For this review, take the finished solid that the model builds, in its own axes (mm). A direction names the side the tool comes from. Coordinates: 2 decimals unless noted, no trailing zeros. Write each loop counter-clockwise with the first axis right and the second up, starting at its lowest first coordinate (ties: lowest second). Pieces come first, ordered by that corner, then holes. Notation, with made-up numbers: M 40.25,-32.75 L 74.25,-32.75 A18 ccw 74.25,-17.75 Z; hole C -35.5,-10.75 d7. An arc over 180 degrees is marked long. Return JSON: item names as keys, results as strings.
```python
from build123d import *

# Parameters (mm, degrees)
F2_R     = 3.81
F3_R     = 5.5372
F4_DEPTH = 177.8


with BuildPart() as f1:
    # F0 (on Front) → F1 (revolve)
    with BuildSketch(Plane.XZ):
        Polygon((0, 6.35), (0, 0), (11.811, 0), (12.7, 12.192), (12.446, 12.192), (10.922, 6.35), align=None)
    revolve(axis=Axis((0, 0, 3.175), (0, 0, -1)))

    # F2
    f2_edges = [f1.edges().sort_by_distance(p)[0] for p in [
        (-11.811, 0, 0),
    ]]
    fillet(f2_edges, radius=F2_R)

    # F3 (on face) → F4 (join)
    with BuildSketch(Plane(origin=(0, 0, 0), x_dir=(1, 0, 0), z_dir=(0, 0, -1))):
        Circle(F3_R)
    extrude(amount=F4_DEPTH)


solid = f1.part
```
1. Clearance check with flat-ended pins moving along their axes: pin 1 Ø8 at (y, z) = (7, -81.5) entering from +X; pin 2 Ø2 at (y, z) = (4, -148) entering from -X; pin 3 Ø1.5 at (x, y) = (8.5, -1.5) entering from +Z; pin 4 Ø8 at (x, y) = (-9.5, -6) entering from +Z. State where each tip first meets the part, or that it passes through.
Checks:
{"pin 1": "x = 4.65", "pin 2": "x = -4.65", "pin 3": "z = 6.35", "pin 4": "z = 12.19"}
2. We need section C-C (z = -136.5). State the section outline as (x, y) points.
Checks:
{"outline": "C 0,0 d11.07"}
3. We need section A-A (y = 0). State the section outline as (x, z) points, plus the area to 3 significant figures.
Checks:
{"outline": "M -12.7,12.19 L -12.07,3.53 A3.81 ccw -8.27,0 L -5.54,0 L -5.54,-177.8 L 5.54,-177.8 L 5.54,0 L 8.27,0 A3.81 ccw 12.07,3.53 L 12.7,12.19 L 12.45,12.19 L 10.92,6.35 L -10.92,6.35 L -12.45,12.19 Z", "area": "2,130 mm2"}
4. For faces 4 (the face through (0, 0, -177.8)), 5 (the face through (-4.394, 3.369, -87.655)), 6 (the face through (0, 0, 6.35)), list the 3-axis set-ups (+Z, -Z, +X, -X, +Y, -Y) from which the entire face can be reached by the end or side of a thin tool; tool diameter is ignored.
Checks:
{"face 4": "-Z, +X, -X, +Y, -Y", "face 5": "-Z", "face 6": "+Z"}
5. Draft analysis for pull direction X (two halves, no side actions). For faces 1 (the face through (-5.4, -2, 0)), 2 (the face through (-2.67, 12.026, 6.961)), 3 (the face through (10.49, -3.3, 6.63)), state which applies: +X half, -X half, draft (parallel to the pull), parting line (faces both ways), or undercut.
Checks:
{"face 1": "draft", "face 2": "parting line", "face 3": "undercut"}
6. Wall thickness on L1, parallel to Z at x = -2, y = 3.5; L2, parallel to Z at x = -6.75, y = 1.5; L3, parallel to Y at x = -0.25, z = -111.5: over which ranges is each line inside the solid? List them lowest first. Write a range as from..to.
Checks:
{"L1": "-177.8..6.35", "L2": "0..6.35", "L3": "-5.53..5.53"}
